Model file for the job. Use its own axes, mm. Face numbers are marked on the shaded views. A direction names the side the tool comes from. Coordinates: 2 decimals unless noted, no trailing zeros. Order: outer loops, then holes, each group sorted by start corner. A loop starts at its lowest first (then second) coordinate and runs counter-clockwise, first axis right, second up.
from build123d import *

# Parameters (mm, degrees)
CUT_EXTRUDE1_DEPTH = 12.65
CIRPATTERN1_COUNT  = 26


with BuildPart() as part:
    # Sketch1 → Revolve1 (revolve)
    with BuildSketch(Plane.XY):
        Polygon((-5, 8.02), (5, 8.02), (5, 6), (6.65, 6), (6.65, 4.225), (6.425, 4), (-6.425, 4), (-6.65, 4.225), (-6.65, 6), (-5, 6), align=None)
    revolve(axis=Axis((17.85, 0, 0), (-1, 0, 0)))

    # Sketch5 → Cut-Extrude1 (cut, through all)
    with BuildSketch(Plane(origin=(-5, 0, -21.5), x_dir=(0, 0, 1), z_dir=(-1, 0, 0))):
        with BuildLine():
            Line((19, 7.620393691), (19, 7.888322065))
            ThreePointArc((19, 7.888322065), (21.5, 8.275), (24, 7.888322065))
            Line((24, 7.888322065), (24, 7.620393691))
            ThreePointArc((24, 7.620393691), (23.15727635, 7.846899713), (22.294932233, 7.980506422))
            ThreePointArc((22.294932233, 7.980506422), (22.212418714, 7.955529493), (22.171812608, 7.879480351))
            ThreePointArc((22.171812608, 7.879480351), (21.5, 7.26999997), (20.828187392, 7.879480351))
            ThreePointArc((20.828187392, 7.879480351), (20.787581286, 7.955529493), (20.705067767, 7.980506422))
            ThreePointArc((20.705067767, 7.980506422), (19.84272365, 7.846899713), (19, 7.620393691))
        make_face()
    cut_extrude1 = extrude(amount=-CUT_EXTRUDE1_DEPTH, mode=Mode.SUBTRACT)

    # CirPattern1: Cut-Extrude1 ×26 about axis
    cirpattern1_axis = Axis((0, 0, 0), (1, 0, 0))
    for i in range(1, CIRPATTERN1_COUNT):
        add(cut_extrude1.rotate(cirpattern1_axis, i * 360 / CIRPATTERN1_COUNT), mode=Mode.SUBTRACT)


solid = part.part
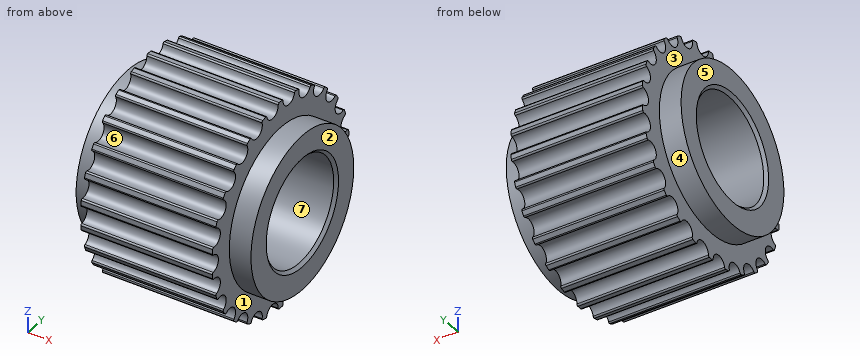
Q1. Cut at B-B, the plane x = 5.75. List the corners of the cut face in (y, z).
Established:
outline: circle Ø12 at (0, 0); hole circle Ø8 at (0, 0)
Q2. Cut at C-C, the plane y = 4.5. List the corners of the cut face in (x, z).
Established:
outline: (-6.65, -3.97) - (-5, -3.97) - (-5, -5.86) - (5, -5.86) - (5, -3.97) - (6.65, -3.97) - (6.65, 3.97) - (5, 3.97) - (5, 5.86) - (-5, 5.86) - (-5, 3.97) - (-6.65, 3.97) - close
Q3. Mould opens along Y. For the marked faces 4, 5, 6 and 7 say: pulls with the +Y half, pulls with the -Y half, needs draft (parallel to the pull), parting line crosses it, or undercut.
Established:
face 4: parting line crosses it
face 5: needs draft
face 6: undercut
face 7: undercut
Q4. Probe line 1 (Z direction, x = 3.5, y = 0); line 2 (Y direction, x = -2.5, z = 0); line 3 (Z direction, x = 2.25, y = -6.5). List the from-to ranges inside material, lowest first.
Established:
line 1: z = -8.02 to -4, 4 to 8.02
line 2: y = -7.27 to -4, 4 to 7.27
line 3: z = -4.7 to -4.1, -3.28 to 3.28, 4.1 to 4.7
Q5. Cut at A-A, the plane z = 0. List the corners of the cut face in (x, y) (3 decimals), plus the area to 3 significant figures.
Established:
outline: (-6.65, -6) - (-5, -6) - (-5, -7.27) - (5, -7.27) - (5, -6) - (6.65, -6) - (6.65, -4.225) - (6.425, -4) - (-6.425, -4) - (-6.65, -4.225) - close; (-6.65, 4.225) - (-6.425, 4) - (6.425, 4) - (6.65, 4.225) - (6.65, 6) - (5, 6) - (5, 7.27) - (-5, 7.27) - (-5, 6) - (-6.65, 6) - close
area: 78.5 mm2
Q6. Which spindle directions (+Z, -Z, +X, -X, +Y, -Y) get a long thin tool onto all of the face, cutting with end or side? Do the marked faces 1, 2 and 3. Say none if no direction does.
Established:
face 1: +X
face 2: +Z, -Z, +X, +Y, -Y
face 3: -X
Q7. Drop a flat-ended pin along its axis: P1, Ø6, axis at x = -4.5, y = -6, coming from the -Z side. Give the stop position or say it passes through.
Established:
P1: stops at z = -7.19
